Source: CAD feature listing. Evaluate the final solid. Frame: model axes, mm. Face numbers are marked on the shaded views. A direction names the side the tool comes from. Give positions to 0.01 mm unless a question says otherwise; leave off trailing zeros. Order: outer loops, then holes, each group sorted by start corner. A loop starts at its lowest first (then second) coordinate and runs counter-clockwise, first axis right, second up. Notation, with made-up numbers: M 18,65 L 23,65 A22 cw 23,75 Z; hole C 10.5,64.25 d5. An arc over 180 degrees is marked long. Answer as a JSON object with one key per item and string values. Group by question number.
1. Pin query (flat end, axial travel): P1, Ø4, axis at x = 55, z = -16.5, coming from the -Y side; P2, Ø5, axis at x = 57, z = 3, coming from the -Y side; P3, Ø10, axis at x = 25.5, z = 44.5, coming from the +Y side. Return the tip coordinate at first contact, or that it passes through.
2. Material intervals for L1, parallel to X at y = 38, z = 25.5 (1 decimal); L2, parallel to Z at x = -89, y = 57.5; L3, parallel to Y at x = 29.5, z = -41.5, sorted ascending. Write a range as [from, to].
3. Section query C-C (z = 36). Output: boundary loops of the cut face in (x, y) (1 decimal).
4. Section query B-B (y = 17). Count the separate pieces of the cut face and the enclosed holes in it, plus the area to 3 significant figures.
5. Section query A-A (x = 60.5). Output: boundary loops of the cut face in (y, z).
6. Pull-direction query (Z, two-part tool) for the marked faces 1, 2 and 3; classes: +Z half, -Z half, draft (parallel to the pull), parting line (faces both ways), or undercut.
7. Set-up query: the marked faces 4, 5 and 6. Return all of +Z, -Z, +X, -X, +Y, -Y with unobstructed straight access to the full face (end or side cutting, diameter ignored); none if empty.
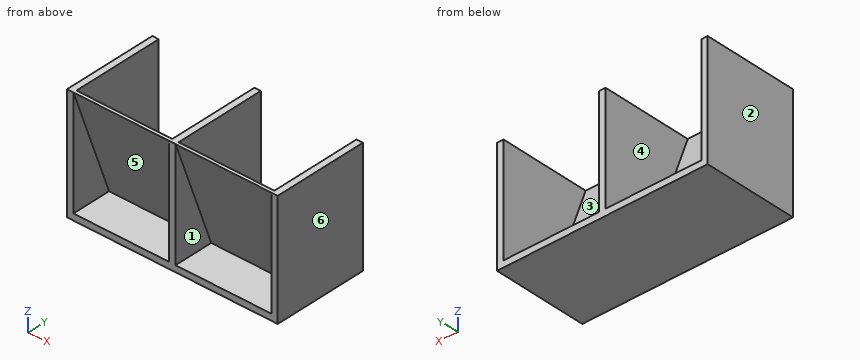
from build123d import *

# Parameters (mm, degrees)
SKETCH1_W            = 209.169
SKETCH1_H            = 114.3
BOX_DEPTH            = 93.98
CUT_EXTRUDE1_REACH   = 153.777
SKETCH2_W            = 95.0595
SKETCH2_H            = 107.95
CUT_EXTRUDE2_START   = -98.2345
CUT_EXTRUDE2_DEPTH   = 95.0595
CUT_EXTRUDE2_START_2 = 3.175
CUT_EXTRUDE2_2_DEPTH = 95.0595


# Read off the part's stored shape, not the designer's step: Cut-Extrude2
with BuildPart() as part:
    # Sketch1 → Box (new body)
    with BuildSketch(Plane(origin=(0, 0, 0), x_dir=(1, 0, 0), z_dir=(0, 1, 0))):
        Rectangle(SKETCH1_W, SKETCH1_H)
    extrude(amount=BOX_DEPTH)

    # Cut-Extrude1: up to this plane
    cut_extrude1_end = Plane(origin=(0, 21.351180018, 7.771193993), z_dir=(0, -0.9396926207859081, -0.34202014332566943))
    # Sketch2 → Cut-Extrude1 (cut, up to the surface)
    with BuildSketch(Plane(origin=(0, 93.98, 0), x_dir=(1, 0, 0), z_dir=(0, 1, 0)), mode=Mode.PRIVATE) as cut_extrude1_sk1:
        with Locations((-50.70475, -3.175)):
            Rectangle(SKETCH2_W, SKETCH2_H)
    cut_extrude1_tool1 = split(extrude(cut_extrude1_sk1.sketch, amount=-CUT_EXTRUDE1_REACH, mode=Mode.PRIVATE), bisect_by=cut_extrude1_end, keep=Keep.BOTH, mode=Mode.PRIVATE)
    add(cut_extrude1_tool1.solids().sort_by_distance((-50.70475, 93.98, 3.175))[0], mode=Mode.SUBTRACT)
    # Sketch2 → Cut-Extrude1 (cut, up to the surface)
    with BuildSketch(Plane(origin=(0, 93.98, 0), x_dir=(1, 0, 0), z_dir=(0, 1, 0)), mode=Mode.PRIVATE) as cut_extrude1_sk2:
        with Locations((50.70475, -3.175)):
            Rectangle(SKETCH2_W, SKETCH2_H)
    cut_extrude1_tool2 = split(extrude(cut_extrude1_sk2.sketch, amount=-CUT_EXTRUDE1_REACH, mode=Mode.PRIVATE), bisect_by=cut_extrude1_end, keep=Keep.BOTH, mode=Mode.PRIVATE)
    add(cut_extrude1_tool2.solids().sort_by_distance((50.70475, 93.98, 3.175))[0], mode=Mode.SUBTRACT)

    # Cut-Extrude2 outline → Cut-Extrude2 (cut)
    with BuildSketch(Plane.YZ.offset(CUT_EXTRUDE2_START)):
        Polygon((0, 57.15), (0, -50.8), (39.290586789, -50.8), align=None)
    extrude(amount=CUT_EXTRUDE2_DEPTH, mode=Mode.SUBTRACT)

    # Cut-Extrude2 2 outline → Cut-Extrude2 2 (cut)
    with BuildSketch(Plane.YZ.offset(CUT_EXTRUDE2_START_2)):
        Polygon((0, 57.15), (0, -50.8), (39.290586789, -50.8), align=None)
    extrude(amount=CUT_EXTRUDE2_2_DEPTH, mode=Mode.SUBTRACT)


solid = part.part
Answer sheet:
{
 "1": {"P1": "y = 26.08", "P2": "y = 18.8", "P3": "y = 9.8"},
 "2": {"L1": "[-104.6, -98.2], [-3.2, 3.2], [98.2, 104.6]", "L2": "[-57.15, -50.8]", "L3": "[35.91, 39.28]"},
 "3": {"outline": "M -104.6,0 L -98.2,0 L -98.2,7.7 L -3.2,7.7 L -3.2,0 L 3.2,0 L 3.2,7.7 L 98.2,7.7 L 98.2,0 L 104.6,0 L 104.6,94 L 98.2,94 L 98.2,11.1 L 3.2,11.1 L 3.2,94 L -3.2,94 L -3.2,11.1 L -98.2,11.1 L -98.2,94 L -104.6,94 Z"},
 "4": {"separate pieces": "1", "enclosed holes": "2", "area": "5,150 mm^2"},
 "5": {"outline": "M 0,-57.15 L 93.98,-57.15 L 93.98,-50.8 L 42.67,-50.8 L 3.38,57.15 L 0,57.15 L 39.29,-50.8 L 0,-50.8 Z"},
 "6": {"face 1": "undercut", "face 2": "draft", "face 3": "+Z half"},
 "7": {"face 4": "+Z, +Y", "face 5": "-Y", "face 6": "+Z, -Z, +X, +Y, -Y"}
}
